Read the model definition and answer for the solid it produces. Units are mm, in the model's axes. A direction names the side the tool comes from. Give positions to 0.01 mm unless a question says otherwise; leave off trailing zeros. Order: outer loops, then holes, each group sorted by start corner. A loop starts at its lowest first (then second) coordinate and runs counter-clockwise, first axis right, second up. Notation, with made-up numbers: (41, 35.5) - (96, 35.5) arc R20 cw to (96, 59.5) - close; hole circle Ø3 at (23, 36.25). An arc over 180 degrees is marked (long way). Return JSON: item names as keys, results as strings.
```python
from build123d import *

# Parameters (mm, degrees)
BASE_EXTRUDE_DEPTH = 101.6
HOLE1_START        = -18.669
HOLE1_OUTLINE_R    = 7.14375
HOLE1_DEPTH        = 1.4986
LPATTERN2_COUNT    = 2
LPATTERN2_PITCH    = 47.625


# Read off the part's stored shape, not the designer's step: Hole1
with BuildPart() as part:
    # Sketch1 → Base-Extrude (new body)
    with BuildSketch(Plane.XY):
        with BuildLine():
            Line((-20.6375, 21.1074), (-20.6375, 11.73965134))
            ThreePointArc((-20.6375, 11.73965134), (-19.1389, 9.144), (-20.6375, 6.54834866))
            Line((-20.6375, 6.54834866), (-20.6375, -6.54834866))
            ThreePointArc((-20.6375, -6.54834866), (-19.1389, -9.144), (-20.6375, -11.73965134))
            Line((-20.6375, -11.73965134), (-20.6375, -17.1704))
            ThreePointArc((-20.6375, -17.1704), (-20.198570222, -18.230070222), (-19.1389, -18.669))
            Line((-19.1389, -18.669), (19.1389, -18.669))
            ThreePointArc((19.1389, -18.669), (20.198570222, -18.230070222), (20.6375, -17.1704))
            Line((20.6375, -17.1704), (20.6375, -11.73965134))
            ThreePointArc((20.6375, -11.73965134), (19.1389, -9.144), (20.6375, -6.54834866))
            Line((20.6375, -6.54834866), (20.6375, 6.54834866))
            ThreePointArc((20.6375, 6.54834866), (19.1389, 9.144), (20.6375, 11.73965134))
            Line((20.6375, 11.73965134), (20.6375, 21.1074))
            ThreePointArc((20.6375, 21.1074), (20.198570222, 22.167070222), (19.1389, 22.606))
            Line((19.1389, 22.606), (12.6111, 22.606))
            ThreePointArc((12.6111, 22.606), (11.551429778, 22.167070222), (11.1125, 21.1074))
            Line((11.1125, 21.1074), (11.1125, 16.256))
            Line((11.1125, 16.256), (12.6111, 16.256))
            Line((12.6111, 16.256), (12.6111, 21.1074))
            Line((12.6111, 21.1074), (19.1389, 21.1074))
            Line((19.1389, 21.1074), (19.1389, 12.494971471))
            ThreePointArc((19.1389, 12.494971471), (17.6403, 9.144), (19.1389, 5.793028529))
            Line((19.1389, 5.793028529), (19.1389, -5.793028529))
            ThreePointArc((19.1389, -5.793028529), (17.6403, -9.144), (19.1389, -12.494971471))
            Line((19.1389, -12.494971471), (19.1389, -17.1704))
            Line((19.1389, -17.1704), (-19.1389, -17.1704))
            Line((-19.1389, -17.1704), (-19.1389, -12.494971471))
            ThreePointArc((-19.1389, -12.494971471), (-17.6403, -9.144), (-19.1389, -5.793028529))
            Line((-19.1389, -5.793028529), (-19.1389, 5.793028529))
            ThreePointArc((-19.1389, 5.793028529), (-17.6403, 9.144), (-19.1389, 12.494971471))
            Line((-19.1389, 12.494971471), (-19.1389, 21.1074))
            Line((-19.1389, 21.1074), (-12.6111, 21.1074))
            Line((-12.6111, 21.1074), (-12.6111, 16.256))
            Line((-12.6111, 16.256), (-11.1125, 16.256))
            Line((-11.1125, 16.256), (-11.1125, 21.1074))
            ThreePointArc((-11.1125, 21.1074), (-11.551429778, 22.167070222), (-12.6111, 22.606))
            Line((-12.6111, 22.606), (-19.1389, 22.606))
            ThreePointArc((-19.1389, 22.606), (-20.198570222, 22.167070222), (-20.6375, 21.1074))
        make_face()
    extrude(amount=BASE_EXTRUDE_DEPTH)

    # Hole1 outline → Hole1 (cut)
    with BuildSketch(Plane(origin=(0, 0, 0), x_dir=(1, 0, 0), z_dir=(0, 1, 0)).offset(HOLE1_START)):
        with Locations((0, -23.8125)):
            Circle(HOLE1_OUTLINE_R)
    hole1 = extrude(amount=HOLE1_DEPTH, mode=Mode.SUBTRACT)

    # LPattern2: Hole1 ×2
    with Locations(*[(0, 0, i * LPATTERN2_PITCH) for i in range(1, LPATTERN2_COUNT)]):
        add(hole1, mode=Mode.SUBTRACT)


solid = part.part
```
Q1. For faces 1 (the flat face through (-20.638, -14, 50)), 2 (the flat face through (19.139, 17, 50)), determine the directions among +Z, -Z, +X, -X, +Y, -Y from which every point of the face is accessible in a straight line to the end or side of a thin tool.
Values:
{"face 1": "+Z, -Z, -X, +Y, -Y", "face 2": "+Z, -Z"}
Q2. A cutting plane is placed at B-B (y = -1.5). Write down the section's boundary in (x, z).
Values:
{"outline": "(-20.64, 0) - (-19.14, 0) - (-19.14, 101.6) - (-20.64, 101.6) - close; (19.14, 0) - (20.64, 0) - (20.64, 101.6) - (19.14, 101.6) - close"}
Q3. A cutting plane is placed at A-A (x = 0). Write down the section's boundary in (y, z).
Values:
{"outline": "(-18.67, 0) - (-17.17, 0) - (-17.17, 16.67) - (-18.67, 16.67) - close; (-18.67, 30.96) - (-17.17, 30.96) - (-17.17, 64.29) - (-18.67, 64.29) - close; (-18.67, 78.58) - (-17.17, 78.58) - (-17.17, 101.6) - (-18.67, 101.6) - close"}
Q4. Given pin 1 (8.5 mm diameter, centred on x = 0, z = 71.44, fed in from +Y); pin 2 (19 mm diameter, centred on x = 2, z = 67, fed in from +Y), each flat-ended and moving along its own axis, determine where each tip first touches the part or whether it passes through.
Values:
{"pin 1": "passes through", "pin 2": "stops at y = 22.11"}
Q5. Determine the mould class of faces 3 (the cylindrical face through (-1.549, -17.93, 30.786)), 4 (the flat face through (20.638, 16, 50)), 5 (the flat face through (0, -18, 0)), 6 (the flat face through (0, -18, 101.6)) for opening direction Z: released by +Z, released by -Z, zero draft, split by the parting line, or undercut.
Values:
{"face 3": "undercut", "face 4": "zero draft", "face 5": "released by -Z", "face 6": "released by +Z"}
Q6. A cutting plane is placed at C-C (y = -7.5). Write down the section's boundary in (x, z), and give its area (3 significant figures).
Values:
{"outline": "(-19.63, 0) - (-17.95, 0) - (-17.95, 101.6) - (-19.63, 101.6) - close; (17.95, 0) - (19.63, 0) - (19.63, 101.6) - (17.95, 101.6) - close", "area": "341 mm²"}
Q7. Consider L1, parallel to Z at x = 0, y = -18.1; L2, parallel to X at y = 17, z = 22.5; L3, parallel to X at y = 0.5, z = 21.5. Determine where each line is inside the solid, lowest interval first.
Values:
{"L1": "z = 0 to 16.67, 30.96 to 64.29, 78.58 to 101.6", "L2": "x = -20.64 to -19.14, -12.61 to -11.11, 11.11 to 12.61, 19.14 to 20.64", "L3": "x = -20.64 to -19.14, 19.14 to 20.64"}
